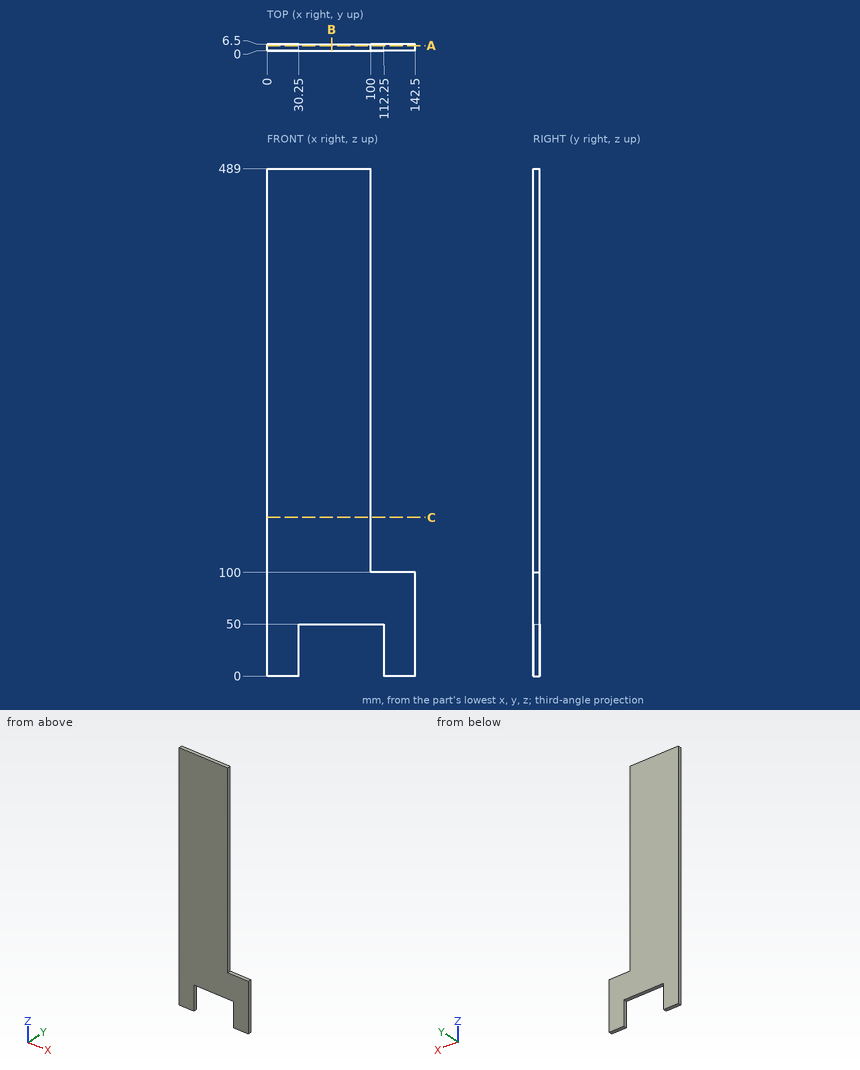
Design review of the part shown in the three views and the two pictorial views. Dimensions are in mm from the part's minimum x, y and z. Give positions to 0.01 mm unless a question says otherwise; leave off trailing zeros. Loops run counter-clockwise (first coordinate to the right, second up) from the corner with the lowest first, then second, coordinate; pieces in that order, holes last. Notation, with made-up numbers: M -25,4.5 L 26,4.5 A28 cw 26,28.5 Z; hole C 36,-35.75 d7. An arc over 180 degrees is marked long. Write item = value, one per line.
Q1. We need section C-C (z = 153). Give the boundary of the cut face in (x, y), plus the area to 3 significant figures.
Output values:
outline = M 0,0 L 100,0 L 100,6.5 L 0,6.5 Z
area = 650 mm^2
Q2. To check wall thickness, follow line 1 (Z direction, x = 35, y = 6); line 2 (X direction, y = 6, z = 297). State the ranges of each line that lie inside material, in increasing order. Write a range as [from, to].
Output values:
line_1 = [50, 489]
line_2 = [0, 100]
Q3. We need section B-B (x = 62). Give the boundary of the cut face in (y, z), plus the area to 3 significant figures.
Output values:
outline = M 0,50 L 6.5,50 L 6.5,489 L 0,489 Z
area = 2,850 mm^2
Q4. We need section A-A (y = 5). Give the boundary of the cut face in (x, z).
Output values:
outline = M 0,0 L 30.25,0 L 30.25,50 L 112.25,50 L 112.25,0 L 142.5,0 L 142.5,100 L 100,100 L 100,489 L 0,489 Z
Q5. Insertion check: pin 1 (2 mm diameter, centred on x = 81, z = 283.5, fed in from -Y); pin 2 (3 mm diameter, centred on x = 119, y = 4.5, fed in from +Z); pin 3 (3 mm diameter, centred on y = 3, z = 356.5, fed in from +X). Each pin has a flat end and moves straight along its axis. Give the tip position at first contact, or say it passes through.
Output values:
pin_1 = 0
pin_2 = 100
pin_3 = 100
